Build history of the part. All positions in model axes, mm. Round coordinates to 2 decimals unless told otherwise and drop trailing zeros. Write each loop counter-clockwise with the first axis right and the second up, starting at its lowest first coordinate (ties: lowest second). Pieces come first, ordered by that corner, then holes. Notation, with made-up numbers: M 59,58 L 64,58 A15 ccw 64,85 Z; hole C 77.5,4.5 d6. An arc over 180 degrees is marked long. Write item = value, one per line.
Autodesk Inventor part; units mm, degrees
ref_plane "YZ Plane" through (0, 0, 0) normal (1, 0, 0) x (0, 1, 0)
ref_plane "XZ Plane" through (0, 0, 0) normal (0, 1, 0) x (-1, 0, 0)
ref_plane "XY Plane" through (0, 0, 0) normal (0, 0, 1) x (1, 0, 0)
sketch "Sketch1" plane through (0, 0, 0) normal (0, 1, 0) x (-1, 0, 0)
  circle A0 centre (-24.5, -25) radius 1.5
  circle A1 centre (-24.5, 25) radius 1.5
  circle A2 centre (22.5, 25) radius 1.5
  circle A3 centre (22.5, -25) radius 1.5
  line L0 (-27.5, -28) -> (-8, -28)
  line L1 (-8, -28) -> (-8, -25) construction
  line L2 (6, -25) -> (6, -28) construction
  line L3 (6, -28) -> (25.5, -28)
  line L4 (25.5, -28) -> (25.5, 28)
  line L5 (25.5, 28) -> (6, 28)
  line L6 (-8, 28) -> (-27.5, 28)
  line L7 (-27.5, 28) -> (-27.5, 39.1)
  arc A4 (-27.5, 39.1) -> (-27.5, -39.1) centre (-22.3277, 0) ccw
  line L8 (-27.5, -39.1) -> (-27.5, -28)
  line L9 (-8, 28) -> (6, 28)
  line L10 (-8, -25) -> (-8, 28) construction
  line L11 (6, -25) -> (6, 28) construction
  line L12 (-8, -28) -> (6, -28)
  line L13 (22.75, 28) -> (-24.75, 28) construction
  line L14 (-24.75, 22) -> (22.75, 22) construction
  line L15 (25.5, -22) -> (-24.75, -22) construction
  line L16 (-24.75, -28) -> (22.75, -28) construction
  line L17 (-8, 28) -> (-27.5, 28) construction
  line L18 (-27.5, 28) -> (-27.5, 39.1) construction
  arc A5 (-27.5, 39.1) -> (-27.5, -39.1) centre (-22.3277, 0) ccw construction
  circle A6 centre (-38.9568, 20.5358) radius 1
  line L19 (-40.0897, 25.2111) -> (-34.2841, 19.3919)
  line L20 (-46.4612, 18.8546) -> (-40.0897, 25.2111)
  circle A7 centre (-41.7885, 17.7107) radius 1
  line L21 (-46.4612, 18.8546) -> (-40.6556, 13.0354)
  line L22 (-34.2841, 19.3919) -> (-40.6556, 13.0354)
  line L23 (-39.9854, 35.3107) -> (-39.9038, 35.3078) construction
  circle A8 centre (-34.6947, 32.6244) radius 1
  line L24 (-39.0291, 26.2718) -> (-38.7163, 35.2301)
  circle A9 centre (-34.8343, 28.6268) radius 1
  line L25 (-39.0291, 26.2718) -> (-30.8141, 25.9849)
  line L26 (-30.5, 34.9794) -> (-30.8141, 25.9849)
  circle A10 centre (-50.0144, 13.6765) radius 1
  line L27 (-47.5144, 9.5665) -> (-47.5144, 17.7865)
  circle A11 centre (-54.0144, 13.6765) radius 1
  line L28 (-56.5144, 17.7865) -> (-47.5144, 17.7865)
  line L29 (-56.5144, 9.5665) -> (-56.5144, 17.7865)
  line L30 (-47.5144, 9.5665) -> (-56.5144, 9.5665)
  line L31 (-39.0291, 26.2718) -> (-67.0612, -1.7603) construction
  line L32 (-39.0291, 26.2718) -> (0.6143, 26.2718) construction
  line L33 (-38.7163, 35.2301) -> (-30.5, 34.9794)
  line L34 (-27.5, -28) -> (-27.5, -22) construction
  line L35 (-27.5, -22) -> (-24.75, -22) construction
  line L36 (-27.5, 28) -> (-27.5, 22) construction
  line L37 (-24.75, 22) -> (-27.5, 22) construction
  line L38 (-27.5, 22) -> (-27.5, 28) construction
  line L39 (-27.5, -22) -> (-27.5, -28) construction
  point P0 (0, 0)
  point P1 (0, 0)
  point P2 (-1, 28)
  point P3 (-1, -22)
  point P4 (-1, -28)
  point P5 (0, 0)
  point P6 (4.5, 0)
  dimension "d0" = 47.5
  dimension "d1" = 6
  dimension "d3" = 47.5
  dimension "d4" = 6
  dimension "d8" = 39.4406
  dimension "d9" = 5.1723
  dimension "d10" = 3
  dimension "d11" = 3
  dimension "d12" = 3
  dimension "d13" = 3
  dimension "d14" = 2
  dimension "d15" = 2
  dimension "d16" = 135
  dimension "d17" = 178
  dimension "d18" = 180
  dimension "d19" = 1.5
  dimension "d20" = 1.5
  dimension "d21" = 1.7282
  dimension "d22" = 8.22
  dimension "d23" = 9
  dimension "d24" = 2
  dimension "d25" = 2
  dimension "d26" = 2.5
  dimension "d27" = 4.11
  dimension "d28" = 4.11
  dimension "d29" = 2.5
  dimension "d30" = 8.22
  dimension "d31" = 2.5
  dimension "d32" = 9
  dimension "d33" = 2.5
  dimension "d34" = 4.11
  dimension "d35" = 4.11
  dimension "d36" = 9
  dimension "d37" = 8.22
  dimension "d38" = 4.11
  dimension "d39" = 2.5
  dimension "d40" = 2.5
  dimension "d41" = 4.11
  dimension "d42" = 3
  dimension "d58" = 3
  dimension "d59" = 53
  dimension "d60" = 3
  dimension "d61" = 3
  dimension "d62" = 3
extrude "Extrusion1" add sketch "Sketch1" along normal blind 1.75 contours L8 A4 L7 L6 L9 L5 L4 L3 L12 L0 | A6 | L19 L22 L21 L20 | A7 | A8 | L24 L33 L26 L25 | A9 | A10 | L30 L29 L28 L27 | A11
sketch "Sketch2" plane through (0, 0, 0) normal (0, -1, 0) x (1, 0, 0)
  circle A0 centre (-17.5, -25) radius 1.5
  circle A1 centre (-17.5, 25) radius 1.5
  circle A2 centre (19.5, 25) radius 1.5
  circle A3 centre (19.5, -25) radius 1.5
  line L0 (27.5, -28) -> (-25.5, -28)
  line L1 (27.5, -39.1) -> (27.5, -28)
  arc A4 (27.5, 39.1) -> (27.5, -39.1) centre (22.3277, 0) ccw
  line L2 (27.5, 28) -> (27.5, 39.1)
  line L3 (-25.5, 28) -> (27.5, 28)
  line L4 (-25.5, -28) -> (-25.5, 28)
  line L5 (24.75, 28) -> (-22.75, 28)
  line L6 (-22.75, 28) -> (-22.75, 22)
  line L7 (-22.75, 22) -> (24.75, 22)
  line L8 (24.75, 22) -> (24.75, 28)
  line L9 (24.75, -22) -> (-22.75, -22)
  line L10 (-22.75, -22) -> (-22.75, -28)
  line L11 (-22.75, -28) -> (24.75, -28)
  line L12 (24.75, -28) -> (24.75, -22)
  point P0 (0, 0)
  point P1 (1, 28)
  point P2 (1, -28)
  dimension "d45" = 47.5
  dimension "d46" = 6
  dimension "d48" = 5.25
  dimension "d49" = 5.25
  dimension "d50" = 47.5
  dimension "d51" = 6
  dimension "d52" = 5.25
  dimension "d53" = 5.25
extrude "Extrusion2" cut sketch "Sketch1" along normal blind 0.1 contours L19 L22 L21 L20 | L24 L33 L26 L25 | L30 L29 L28 L27
mirror "Mirror1" about plane through (0, 0, 0) normal (0, 0, 1) of "Extrusion2"
properties part number "PCB_final"
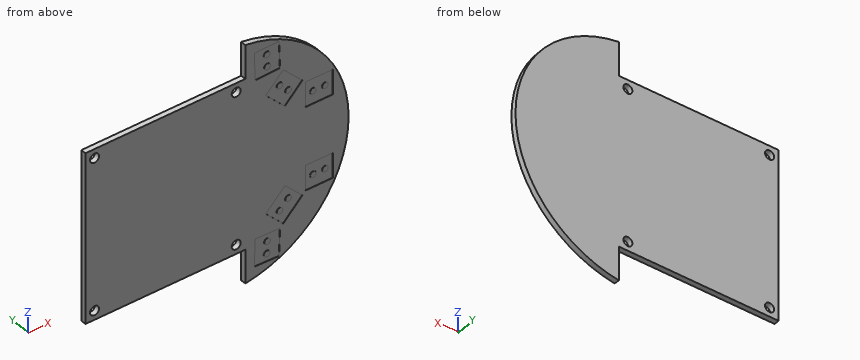
1. Probe probe 1 along Z at (x, y) = (-22.5, 0.5); probe 2 along Z at (x, y) = (-9, 1.1); probe 3 along Y at (x, z) = (48.5, 16). List the from-to ranges inside material, lowest first.
Responses:
probe_1 = -28 to -26.5, -23.5 to 23.5, 26.5 to 28
probe_2 = -28 to 28
probe_3 = 0.1 to 1.75
2. Band-saw the part on B-B (y = 0.9). List the corners of the cut face in (x, z).
Responses:
outline = M -25.5,-28 L 27.5,-28 L 27.5,-39.1 A39.44 ccw 27.5,39.1 L 27.5,28 L -25.5,28 Z; hole C -22.5,-25 d3; hole C -22.5,25 d3; hole C 24.5,-25 d3; hole C 24.5,25 d3
3. Flat gauge pins, fed straight in: pin 1 (1 mm diameter, centred on y = 0.5, z = 3.5, fed in from +X); pin 2 (0.9 mm diameter, centred on y = 1, z = -35, fed in from -X); pin 3 (0.5 mm diameter, centred on x = 13.5, y = 1, fed in from -Z). Where does each tip first touch, or does it go through?
Responses:
pin_1 = 61.65
pin_2 = 27.5
pin_3 = -28
4. Band-saw the part on A-A (x = 24.5). List the corners of the cut face in (y, z), plus the area to 3 significant figures.
Responses:
outline = M 0,-28 L 1.75,-28 L 1.75,-26.5 L 0,-26.5 Z; M 0,-23.5 L 1.75,-23.5 L 1.75,23.5 L 0,23.5 Z; M 0,26.5 L 1.75,26.5 L 1.75,28 L 0,28 Z
area = 87.5 mm²
